from build123d import *

# Parameters (mm, degrees)
SKETCH1_W           = 504
SKETCH1_H           = 504
BOSS_EXTRUDE1_DEPTH = 205
SKETCH2_W           = 500
SKETCH2_H           = 500
CUT_EXTRUDE1_DEPTH  = 200
FILLET2_R           = 10
FILLET4_R           = 10


with BuildPart() as part:
    # Sketch1 → Boss-Extrude1 (new body)
    with BuildSketch(Plane.XY):
        Rectangle(SKETCH1_W, SKETCH1_H)
    extrude(amount=BOSS_EXTRUDE1_DEPTH)

    # Sketch2 → Cut-Extrude1 (cut)
    with BuildSketch(Plane(origin=(0, 0, 0), x_dir=(-1, 0, 0), z_dir=(0, 0, -1))):
        Rectangle(SKETCH2_W, SKETCH2_H)
    extrude(amount=-CUT_EXTRUDE1_DEPTH, mode=Mode.SUBTRACT)

    # Fillet2
    # the kernel refuses this fillet: 10 mm, written as the material it adds along each edge
    with BuildSketch(Plane(origin=(-250, -250, 0), x_dir=(0, 1, 0), z_dir=(0, 0, 1))) as fillet2_piece_1:
        with BuildLine():
            CenterArc((FILLET2_R, -FILLET2_R), FILLET2_R, 90, 90)
            Line((0, -FILLET2_R), (0, 0))
            Line((0, 0), (FILLET2_R, 0))
        make_face()
    extrude(amount=200)
    # the kernel refuses this fillet: 10 mm, written as the material it takes off along each edge
    with BuildSketch(Plane(origin=(-277, -252, 0), x_dir=(0, 1, 0), z_dir=(1, 0, 0))) as fillet2_2_piece_1:
        with BuildLine():
            CenterArc((FILLET2_R, FILLET2_R), FILLET2_R, 180, 90)
            Line((0, FILLET2_R), (0, 0))
            Line((0, 0), (FILLET2_R, 0))
        make_face()
    extrude(amount=554, mode=Mode.SUBTRACT)
    with BuildSketch(Plane(origin=(252, -277, 0), x_dir=(0, 0, 1), z_dir=(0, 1, 0)), Plane(origin=(277, 252, 0), x_dir=(0, 0, 1), z_dir=(-1, 0, 0)), Plane(origin=(-252, 277, 0), x_dir=(0, 0, 1), z_dir=(0, -1, 0))) as fillet2_2_piece_2:
        with BuildLine():
            CenterArc((FILLET2_R, -FILLET2_R), FILLET2_R, 90, 90)
            Line((0, -FILLET2_R), (0, 0))
            Line((0, 0), (FILLET2_R, 0))
        make_face()
    extrude(amount=554, mode=Mode.SUBTRACT)

    # Fillet4
    fillet4_edges = [part.edges().sort_by_distance(p)[0] for p in [
        (5, -250, 200),
        (250, 0, 200),
        (0, 250, 200),
        (-250, 5, 200),
        (-247.071067812, -247.071067812, 200),
    ]]
    fillet(fillet4_edges, radius=FILLET4_R)


solid = part.part
Build history of the part. All positions in model axes, mm. A direction names the side the tool comes from. Round coordinates to 2 decimals unless told otherwise and drop trailing zeros. Loops run counter-clockwise (first coordinate to the right, second up) from the corner with the lowest first, then second, coordinate; pieces in that order, holes last. Notation, with made-up numbers: (88.5, 82.5) -> (105.5, 82.5) arc R18 ccw to (105.5, 102.5) -> close; hole circle Ø7 at (-8.75, 40). An arc over 180 degrees is marked (long way). One line per item, written item: value. Start each with the question number.
Q1. Drop a flat-ended pin along its axis: pin 1 Ø1 at (x, y) = (183, -201.5) entering from -Z. Give the stop position or say it passes through.
Q2. Cut at A-A on z = 65. List the corners of the cut face in (x, y), plus the area to 3 significant figures.
Q3. Two-plate mould, pull along Y, no slides. Class faces 1 (the face through (-4, 252, 106)), 2 (the face through (3, 3, 200)), 3 (the face through (-252, -4, 106)): released by +Y, released by -Y, zero draft, split by the parting line, or undercut.
Q4. 3-axis set-ups, long thin cutter, end or side, ignore diameter. For faces 4 (the face through (-4, 4, 205)), 5 (the face through (250, -3, 96)): which of +Z, -Z, +X, -X, +Y, -Y reach the whole face in a straight line?
Q5. Cut at B-B on y = -76. List the corners of the cut face in (x, z).
Q6. Probe line 1 along X through (y, z) = (-213, 68.5); line 2 along Y through (x, z) = (-196, 191.5). List the from-to ranges inside material, lowest first.
Computed:
1. pin 1: z = 200
2. outline: (-252, -252) -> (252, -252) -> (252, 252) -> (-252, 252) -> close; hole (-250, -240) arc R10 ccw to (-240, -250) -> (250, -250) -> (250, 250) -> (-250, 250) -> close
2. area: 4,040 mm²
3. face 1: released by +Y
3. face 2: undercut
3. face 3: zero draft
4. face 4: +Z, +X, -X, +Y, -Y
4. face 5: -Z
5. outline: (-252, 10) arc R10 ccw to (-250, 4) -> (-250, 190) arc R10 cw to (-240, 200) -> (240, 200) arc R10 cw to (250, 190) -> (250, 4) arc R10 ccw to (252, 10) -> (252, 205) -> (-252, 205) -> close
6. line 1: -252 to -250, 250 to 252
6. line 2: -252 to -249.89, 249.89 to 252
